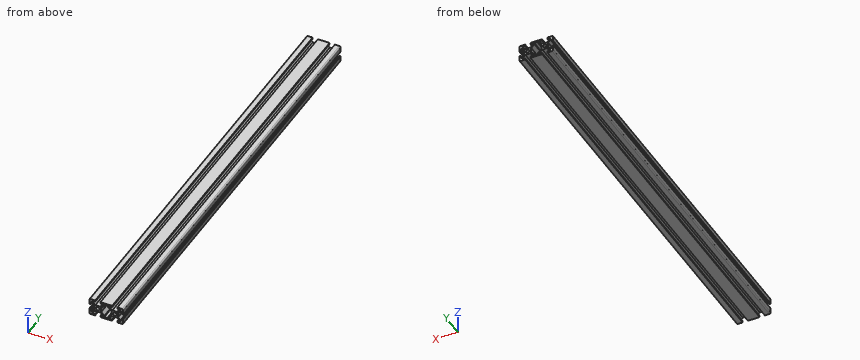
from build123d import *

# Parameters (mm, degrees)
SKETCH_R  = 2.1
PAD_DEPTH = 250
FILLET_R  = 1.5


with BuildPart() as part:
    # Sketch → Pad (new body, symmetric)
    with BuildSketch(Plane.XZ):
        Polygon((-10, 10), (-3.1, 10), (-3.1, 8.2), (-6, 8.2), (-6, 7.06066), (-2.83934, 3.9), (2.83934, 3.9), (6, 7.06066), (6, 8.2), (3.1, 8.2), (3.1, 10), (16.9, 10), (16.9, 8.2), (14, 8.2), (14, 7.06066), (17.16066, 3.9), (22.83934, 3.9), (26, 7.06066), (26, 8.2), (23.1, 8.2), (23.1, 10), (30, 10), (30, 3.1), (28.2, 3.1), (28.2, 6), (27.06066, 6), (23.9, 2.83934), (23.9, -2.83934), (27.06066, -6), (28.2, -6), (28.2, -3.1), (30, -3.1), (30, -10), (23.1, -10), (23.1, -8.2), (26, -8.2), (26, -7.06066), (22.83934, -3.9), (17.16066, -3.9), (14, -7.06066), (14, -8.2), (16.9, -8.2), (16.9, -10), (3.1, -10), (3.1, -8.2), (6, -8.2), (6, -7.06066), (2.83934, -3.9), (-2.83934, -3.9), (-6, -7.06066), (-6, -8.2), (-3.1, -8.2), (-3.1, -10), (-10, -10), (-10, -3.1), (-8.2, -3.1), (-8.2, -6), (-7.06066, -6), (-3.9, -2.83934), (-3.9, 2.83934), (-7.06066, 6), (-8.2, 6), (-8.2, 3.1), (-10, 3.1), align=None)
        Circle(SKETCH_R, mode=Mode.SUBTRACT)
        with Locations((20, 0)):
            Circle(SKETCH_R, mode=Mode.SUBTRACT)
        Polygon((7.8, -6.53934), (4.1, -2.83934), (4.1, 2.83934), (7.8, 6.53934), (7.8, 8.2), (12.2, 8.2), (12.2, 6.53934), (15.9, 2.83934), (15.9, -2.83934), (12.2, -6.53934), (12.2, -8.2), (7.8, -8.2), align=None, mode=Mode.SUBTRACT)
    extrude(amount=PAD_DEPTH, both=True)

    # Fillet
    fillet_edges = [part.edges().sort_by_distance(p)[0] for p in [
        (-10, 0, 10),
        (30, 0, 10),
        (30, 0, -10),
        (-10, 0, -10),
    ]]
    fillet(fillet_edges, radius=FILLET_R)


with BuildPart() as part_1:
    # Body placement: moved
    add(part.part.moved(Location((-30, 0, 0))))


solid = part_1.part
CAD build for the part. Positions are in the model's coordinates, mm. Round coordinates to 2 decimals unless told otherwise and drop trailing zeros. Put each result on its own line as item: value.
1. Pin check, flat tips, straight feed: P1, Ø1.7, axis at y = -96, z = -1, coming from the -X side; P2, Ø0.5, axis at y = 124, z = 9.5, coming from the +X side; P3, Ø3, axis at x = -9.5, y = 94, coming from the +Z side. Stop position of each tip, or through.
Geometry check:
P1: x = -33.9
P2: x = -0.2
P3: z = 3.9
2. Wall check: line 1 (X direction, y = 15, z = 0.5); line 2 (X direction, y = 223, z = -8); line 3 (Z direction, x = -19.5, y = 136). Give the ranges that are in metal, low to high.
Geometry check:
line 1: -33.9 to -32.04, -27.96 to -25.9, -14.1 to -12.04, -7.96 to -6.1
line 2: -40 to -36, -24 to -22.2, -17.8 to -16, -4 to 0
line 3: -10 to -8.2, 8.2 to 10
3. Slice it at A-A on y = -83. Give the number of separate pieces and of enclosed holes in the cut face, and give its area (3 significant figures).
Geometry check:
separate pieces: 1
enclosed holes: 3
area: 312 mm²
